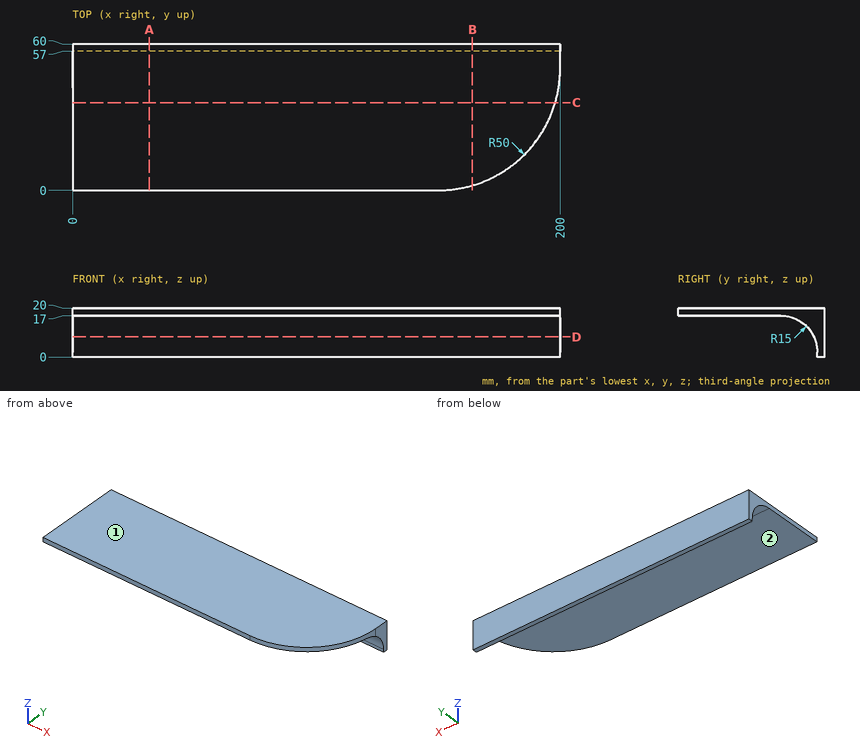
Design review of the part shown in the three views and the two pictorial views. Dimensions are in mm from the part's minimum x, y and z. A direction names the side the tool comes from. Round coordinates to 2 decimals unless told otherwise and drop trailing zeros. Loops run counter-clockwise (first coordinate to the right, second up) from the corner with the lowest first, then second, coordinate; pieces in that order, holes last. Notation, with made-up numbers: M -16,24 L 20,24 A27 ccw 20,42 Z; hole C -14.5,-25.5 d9. An arc over 180 degrees is marked long. Answer as a JSON object with one key per item and string values.
Item 1: We need section B-B on x = 164. Give the boundary of the cut face in (y, z).
Answer sheet:
{"outline": "M 2,17 L 42,17 A15 cw 57,2 L 57,0 L 60,0 L 60,20 L 2,20 Z"}
Item 2: Machinability: for the marked faces 1 and 2, which of the approach directions +Z, -Z, +X, -X, +Y, -Y give a long, thin tool a straight path to every point of the face, cutting with its end or side? Answer none if there is none.
Answer sheet:
{"face 1": "+Z, +X, -X, +Y, -Y", "face 2": "-Z, +X, -X, -Y"}
Item 3: Wall thickness on L1, parallel to Z at x = 44, y = 30; L2, parallel to Y at x = 36, z = 4.25; L3, parallel to Y at x = 81, z = 7.75: over which ranges is each line inside the solid? List them lowest first. Write a range as from..to.
Answer sheet:
{"L1": "z = 17..20", "L2": "y = 56.83..60", "L3": "y = 55.85..60"}
Item 4: We need section D-D on z = 8.25. Give the boundary of the cut face in (x, y), and give its area (3 significant figures).
Answer sheet:
{"outline": "M 0,55.64 L 200,55.64 L 200,60 L 0,60 Z", "area": "873 mm^2"}
Item 5: We need section C-C on y = 36. Give the boundary of the cut face in (x, z).
Answer sheet:
{"outline": "M 0,17 L 198,17 L 198,20 L 0,20 Z"}
Item 6: We need section A-A on x = 31.5. Give the boundary of the cut face in (y, z).
Answer sheet:
{"outline": "M 0,17 L 42,17 A15 cw 57,2 L 57,0 L 60,0 L 60,20 L 0,20 Z"}
Item 7: Clearance check with flat-ended pins moving along their axes: P1, Ø1.6, axis at x = 75.5, z = 0.5, coming from the -Y side; P2, Ø1.5, axis at y = 37, z = 18, coming from the +X side; P3, Ø1.5, axis at x = 121, y = 39.5, coming from the -Z side; P4, Ø5, axis at y = 52.5, z = 4, coming from the +X side. State where each tip first meets the part, or that it passes through.
Answer sheet:
{"P1": "stops at y = 57", "P2": "stops at x = 198.48", "P3": "stops at z = 17", "P4": "passes through"}
